```python
from build123d import *

# Parameters (mm, degrees)
SKETCH_W        = 181.97
SKETCH_H        = 105
SKETCH_R        = 14
SKETCH_R_2      = 2.55
SKETCH_R_3      = 1.75
SKETCH_W_2      = 97.37
SKETCH_H_2      = 39.83
PAD_DEPTH       = 2.5
CHAMFER_SIZE    = 2.2
SKETCH001_R     = 3.5
PAD001_DEPTH    = 4
SKETCH002_R     = 3.5
PAD002_DEPTH    = 5.5
SKETCH003_R     = 2.1
POCKET_DEPTH    = 6
SKETCH004_R     = 1.6
POCKET001_DEPTH = 5.5
FILLET_R        = 4


with BuildPart() as part:
    # Sketch → Pad (new body)
    with BuildSketch(Plane.XY):
        with Locations((90.985, -52.5)):
            Rectangle(SKETCH_W, SKETCH_H)
        with Locations((91.485, -86)):
            Circle(SKETCH_R, mode=Mode.SUBTRACT)
        with Locations((151.485, -86)):
            Circle(SKETCH_R, mode=Mode.SUBTRACT)
        with Locations((136.485, -71)):
            Circle(SKETCH_R_2, mode=Mode.SUBTRACT)
        with Locations((76.485, -71)):
            Circle(SKETCH_R_2, mode=Mode.SUBTRACT)
        with Locations((6, -99)):
            Circle(SKETCH_R_3, mode=Mode.SUBTRACT)
        with Locations((175.97, -99)):
            Circle(SKETCH_R_3, mode=Mode.SUBTRACT)
        with Locations((6, -6)):
            Circle(SKETCH_R_3, mode=Mode.SUBTRACT)
        with Locations((175.97, -6)):
            Circle(SKETCH_R_3, mode=Mode.SUBTRACT)
        with Locations((121.485, -35.17)):
            Rectangle(SKETCH_W_2, SKETCH_H_2, mode=Mode.SUBTRACT)
    extrude(amount=PAD_DEPTH)

    # Chamfer
    chamfer_edges = [part.edges().sort_by_distance(p)[0] for p in [
        (4.25, -6, 2.5),
        (4.25, -99, 2.5),
        (174.22, -99, 2.5),
        (174.22, -6, 2.5),
    ]]
    chamfer(chamfer_edges, length=CHAMFER_SIZE)

    # Sketch001 (on Face3 of Chamfer) → Pad001 (join)
    with BuildSketch(Plane(origin=(0, 0, 0), x_dir=(1, 0, 0), z_dir=(0, 0, -1))):
        with Locations((15.5, 84.3)):
            Circle(SKETCH001_R)
        with Locations((64.5, 84.3)):
            Circle(SKETCH001_R)
        with Locations((64.5, 26.3)):
            Circle(SKETCH001_R)
        with Locations((15.5, 26.3)):
            Circle(SKETCH001_R)
    extrude(amount=PAD001_DEPTH)

    # Sketch002 (on Face3 of Pad001) → Pad002 (join)
    with BuildSketch(Plane(origin=(0, 0, 0), x_dir=(1, 0, 0), z_dir=(0, 0, -1))):
        with Locations((74.985, 63.085)):
            Circle(SKETCH002_R)
        with Locations((167.985, 63.085)):
            Circle(SKETCH002_R)
        with Locations((167.985, 8.085)):
            Circle(SKETCH002_R)
        with Locations((74.985, 8.085)):
            Circle(SKETCH002_R)
    extrude(amount=PAD002_DEPTH)

    # Sketch003 (on Face33 of Pad002) → Pocket (cut)
    with BuildSketch(Plane(origin=(0, 0, -5.5), x_dir=(1, 0, 0), z_dir=(0, 0, -1))):
        with Locations((74.985, 63.085)):
            Circle(SKETCH003_R)
        with Locations((167.985, 63.085)):
            Circle(SKETCH003_R)
        with Locations((167.985, 8.085)):
            Circle(SKETCH003_R)
        with Locations((74.985, 8.085)):
            Circle(SKETCH003_R)
    extrude(amount=-POCKET_DEPTH, mode=Mode.SUBTRACT)

    # Sketch004 (on Face36 of Pocket) → Pocket001 (cut)
    with BuildSketch(Plane(origin=(0, 0, -4), x_dir=(1, 0, 0), z_dir=(0, 0, -1))):
        with Locations((15.5, 84.3)):
            Circle(SKETCH004_R)
        with Locations((64.5, 84.3)):
            Circle(SKETCH004_R)
        with Locations((64.5, 26.3)):
            Circle(SKETCH004_R)
        with Locations((15.5, 26.3)):
            Circle(SKETCH004_R)
    extrude(amount=-POCKET001_DEPTH, mode=Mode.SUBTRACT)

    # Fillet
    fillet_edges = [part.edges().sort_by_distance(p)[0] for p in [
        (0, 0, 1.25),
        (0, -105, 1.25),
        (181.97, 0, 1.25),
        (181.97, -105, 1.25),
    ]]
    fillet(fillet_edges, radius=FILLET_R)


solid = part.part
```
Source: CAD feature listing. Evaluate the final solid. Frame: model axes, mm. A direction names the side the tool comes from. Round coordinates to 2 decimals unless told otherwise and drop trailing zeros. Write each loop counter-clockwise with the first axis right and the second up, starting at its lowest first coordinate (ties: lowest second). Pieces come first, ordered by that corner, then holes. Notation, with made-up numbers: M 15,-8 L 67,-8 A29 cw 67,25 Z; hole C 24.5,-37.75 d11. An arc over 180 degrees is marked long. Use CSV: the item, a comma, the result in double quotes. Start each with the question number.
Q1. Cut plane C-C on x = 147. Output: boundary loops of the cut face in (y, z) (3 decimals), plus the area to 3 significant figures.
Q2. Cut plane D-D on x = 31.5. Output: boundary loops of the cut face in (y, z).
Q3. Cut plane B-B on y = -77. Output: boundary loops of the cut face in (x, z).
Q4. Line query: line 1 (Y direction, x = 64.5, z = -0.05); line 2 (Y direction, x = 64.5, z = 0.4); line 3 (X direction, y = -99, z = 0.2). Output: solid intervals per line, ascending. Write a range as from..to.
Q5. Cut plane A-A on x = 6. Output: boundary loops of the cut face in (y, z), plus the area to 3 significant figures.
Q6. Access query for faces 1 (the face through (15, -84, 1.5)), 2 (the face through (89.66, -72.12, 1.23)). Directions: +Z, -Z, +X, -X, +Y, -Y. A direction counts if a zero-diameter tool reaches every point of the face in a straight line with its end or side. Return the directions, or none.
Q7. Pull-direction query (X, two-part tool) for faces 3 (the face through (64, -84, 1.5)), 4 (the face through (74.9, -60.8, -5.5)); classes: +X half, -X half, draft (parallel to the pull), parting line (faces both ways), or undercut.
Q8. First-contact query: P1, Ø1.3, axis at x = 168.5, y = -63, coming from the -Z side; P2, Ø1.6, axis at x = 16, y = -25.5, coming from the -Z side; P3, Ø3, axis at y = -66, z = -2.5, coming from the +X side. Flat tips, straight axial feed; report the tip coordinate or a pass-through.
Results found:
1,outline,"M -105,0 L -99.262,0 L -99.262,2.5 L -105,2.5 Z; M -72.738,0 L -55.085,0 L -55.085,2.5 L -72.738,2.5 Z; M -15.255,0 L 0,0 L 0,2.5 L -15.255,2.5 Z"
1,area,"96.6 mm^2"
2,outline,"M -105,0 L 0,0 L 0,2.5 L -105,2.5 Z"
3,outline,"M 0,0 L 80.76,0 L 80.76,2.5 L 0,2.5 Z; M 102.21,0 L 140.76,0 L 140.76,2.5 L 102.21,2.5 Z; M 162.21,0 L 181.97,0 L 181.97,2.5 L 162.21,2.5 Z"
4,line 1,"-87.8..-85.9, -82.7..-80.8, -29.8..-27.9, -24.7..-22.8"
4,line 2,"-105..-85.9, -82.7..-27.9, -24.7..0"
4,line 3,"0..4.25, 7.75..86.29, 96.68..146.29, 156.68..174.22, 177.72..181.97"
5,outline,"M -105,0 L -100.75,0 L -100.75,0.3 L -102.95,2.5 L -105,2.5 Z; M -97.25,0 L -7.75,0 L -7.75,0.3 L -9.95,2.5 L -95.05,2.5 L -97.25,0.3 Z; M -4.25,0 L 0,0 L 0,2.5 L -2.05,2.5 L -4.25,0.3 Z"
5,area,"235 mm^2"
6,face 1,"-Z"
6,face 2,"+Z, -Z"
7,face 3,"undercut"
7,face 4,"draft"
8,P1,"z = 0.5"
8,P2,"z = -4"
8,P3,"x = 171.19"
